The model under review builds one solid part; all positions refer to its coordinate system, in mm. Coordinates: 2 decimals unless noted, no trailing zeros. Loops run counter-clockwise (first coordinate to the right, second up) from the corner with the lowest first, then second, coordinate; pieces in that order, holes last. Notation, with made-up numbers: M 26,45.5 L 55,45.5 A6 ccw 55,53.5 Z; hole C -24,21.5 d4. An arc over 180 degrees is marked long. Use one line per item in the form item = value.
```python
from build123d import *

# Parameters (mm, degrees)
SKETCH1_R           = 1.5
BOSS_EXTRUDE1_DEPTH = 4.75


with BuildPart() as part:
    # Sketch1 → Boss-Extrude1 (new body)
    with BuildSketch(Plane.XY):
        with BuildLine():
            Line((-97.529258778, -78.185955787), (-60, -125))
            Line((-60, -125), (-60, -131))
            Line((-60, -131), (60, -131))
            Line((60, -131), (60, -125))
            Line((60, -125), (97.529258778, -78.185955787))
            ThreePointArc((97.529258778, -78.185955787), (0, 125), (-97.529258778, -78.185955787))
        make_face()
        with Locations((-77.781745931, -77.781745931)):
            Circle(SKETCH1_R, mode=Mode.SUBTRACT)
        with Locations((-20, -110)):
            Circle(SKETCH1_R, mode=Mode.SUBTRACT)
        with Locations((20, -110)):
            Circle(SKETCH1_R, mode=Mode.SUBTRACT)
        with Locations((77.781745931, -77.781745931)):
            Circle(SKETCH1_R, mode=Mode.SUBTRACT)
        with Locations((-110, 0)):
            Circle(SKETCH1_R, mode=Mode.SUBTRACT)
        with BuildLine():
            ThreePointArc((93.01577046, -19.314928054), (-95, 0), (93.01577046, 19.314928054))
            add(Edge.make_bspline(
                [(93.01577046, 19.314928054), (93.70285757, 1.722452045), (81.198007465, 0)],
                knots=[0, 0, 0, 1, 1, 1], degree=2))
            add(Edge.make_bspline(
                [(93.01577046, -19.314928054), (93.70285757, -1.722452045), (81.198007465, 0)],
                knots=[0, 0, 0, 1, 1, 1], degree=2))
        make_face(mode=Mode.SUBTRACT)
        with Locations((-77.781745931, 77.781745931)):
            Circle(SKETCH1_R, mode=Mode.SUBTRACT)
        with Locations((110, 0)):
            Circle(SKETCH1_R, mode=Mode.SUBTRACT)
        with Locations((0, 110)):
            Circle(SKETCH1_R, mode=Mode.SUBTRACT)
        with Locations((77.781745931, 77.781745931)):
            Circle(SKETCH1_R, mode=Mode.SUBTRACT)
    extrude(amount=BOSS_EXTRUDE1_DEPTH)


solid = part.part
```
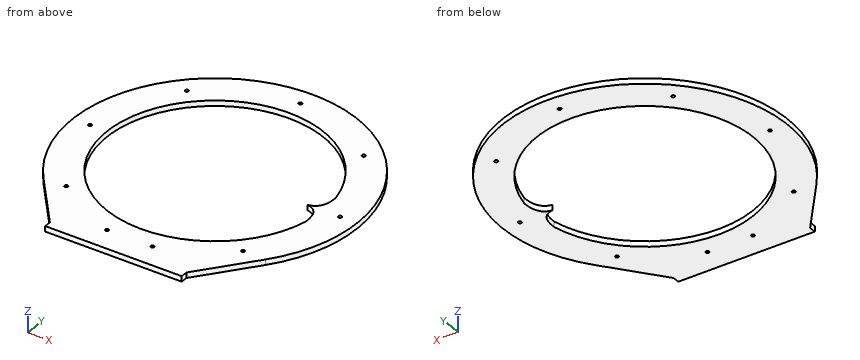
1. Wall thickness on line 1 along Y through (x, z) = (79, 4.5); line 2 along X through (y, z) = (-110, 1.95) (3 decimals); line 3 along Y through (x, z) = (86.5, 4.1): over which ranges is each line inside the solid? List them lowest first. Write a range as from..to.
Response values:
line_1 = -101.3..-78.66, -76.91..-52.76, 52.76..76.91, 78.66..96.87
line_2 = -72.025..-21.5, -18.5..18.5, 21.5..72.025
line_3 = -91.94..-39.28, -1.78..1.78, 39.28..90.24
2. Add section D-D (y = 103). State the section outline as (x, z) points.
Response values:
outline = M -70.82,0 L 70.82,0 L 70.82,4.75 L -70.82,4.75 Z
3. Insertion check: P1, Ø1.8, axis at x = 20, y = -110, coming from the -Z side; P2, Ø1.5, axis at x = 78.5, z = 3.5, coming from the +Y side; P3, Ø2, axis at x = -92.5, z = 1, coming from the +Y side. Each pin has a flat end and moves straight along its axis. Give the tip position at first contact, or say it passes through.
Response values:
P1 = through
P2 = 97.88
P3 = 85.16
4. Add section C-C (z = 1.25). Count the separate pieces of the cut face and the enclosed holes in it, then the cut area to 3 significant figures.
Response values:
separate_pieces = 1
enclosed_holes = 10
area = 22,500 mm^2
5. Add section A-A (x = -52). State the section outline as (y, z) points, then the cut area to 3 significant figures.
Response values:
outline = M -131,0 L -79.5,0 L -79.5,4.75 L -131,4.75 Z; M 79.5,0 L 113.67,0 L 113.67,4.75 L 79.5,4.75 Z
area = 407 mm^2
6. Add section B-B (y = -100). State the section outline as (x, z) points, then the cut area to 3 significant figures.
Response values:
outline = M -80.04,0 L 80.04,0 L 80.04,4.75 L -80.04,4.75 Z
area = 760 mm^2
